Autodesk Inventor part; units mm, degrees
ref_plane "YZ Plane" through (0, 0, 0) normal (1, 0, 0) x (0, 1, 0)
ref_plane "XZ Plane" through (0, 0, 0) normal (0, 1, 0) x (-1, 0, 0)
ref_plane "XY Plane" through (0, 0, 0) normal (0, 0, 1) x (1, 0, 0)
sketch "Sketch1" plane through (0, 0, 0) normal (0, 0, 1) x (1, 0, 0)
  line L0 (-65.0875, -53.975) -> (65.0875, -53.975)
  line L1 (65.0875, -53.975) -> (65.0875, 53.975)
  line L2 (65.0875, 53.975) -> (-65.0875, 53.975)
  line L3 (-65.0875, 53.975) -> (-65.0875, -53.975)
  line L4 (-65.0875, -53.975) -> (65.0875, 53.975) construction
  line L5 (65.0875, -53.975) -> (-65.0875, 53.975) construction
  point P0 (0, 0)
  dimension "d0" = 130.175
  dimension "d1" = 107.95
extrude "Extrusion1" add sketch "Sketch1" along normal blind 209.55
sketch "Sketch2" plane through (0, 0, 209.55) normal (0, 0, 1) x (1, 0, 0)
  line L0 (-65.0875, -53.975) -> (65.0875, -53.975) construction
  line L1 (-65.0875, 53.975) -> (-65.0875, -53.975) construction
  circle A0 centre (-23.8125, -22.225) radius 4
  circle A1 centre (23.8125, 9.525) radius 4
  line L2 (-11.1125, 12.065) -> (-33.3375, 12.065)
  line L3 (-33.3375, 12.065) -> (-33.3375, 13.335)
  line L4 (-33.3375, 13.335) -> (-11.1125, 13.335)
  line L5 (-11.1125, 13.335) -> (-11.1125, 12.065)
  line L6 (-33.3375, 12.7) -> (-65.0875, 12.7) construction
  point P0 (0, 0)
  dimension "d4" = 31.75
  dimension "d5" = 41.275
  dimension "d6" = 8
  dimension "d7" = 63.5
  dimension "d8" = 88.9
  dimension "d13" = 31.75
  dimension "d14" = 53.975
  dimension "d15" = 66.675
  dimension "d16" = 1.27
extrude "Extrusion2" add sketch "Sketch2" along normal blind 12.7
sketch "Sketch3" plane through (0, 0, 0) normal (0, 0, -1) x (-1, 0, 0)
  circle A0 centre (-23.8125, 9.525) radius 4
  circle A1 centre (23.8125, -22.225) radius 4
  line L0 (33.3375, 12.065) -> (11.1125, 12.065)
  line L1 (11.1125, 12.065) -> (11.1125, 13.335)
  line L2 (11.1125, 13.335) -> (33.3375, 13.335)
  line L3 (33.3375, 13.335) -> (33.3375, 12.065)
  point P0 (0, 0)
extrude "Extrusion3" add sketch "Sketch3" along normal blind 12.7
sketch "Sketch4" plane through (-33.3375, 13.335, 0) normal (0, 1, 0) x (1, 0, 0)
  line L0 (0, 12.7) -> (22.225, 12.7)
  line L1 (22.225, 0) -> (22.225, 12.7)
  line L2 (0, 0) -> (0, 12.7)
  line L3 (22.225, -209.55) -> (22.225, -222.25)
  line L4 (22.225, -222.25) -> (0, -222.25)
  line L5 (0, -209.55) -> (0, -222.25)
  line L6 (16.51, -219.71) -> (5.715, -219.71)
  line L7 (5.715, -219.71) -> (5.715, -215.265)
  line L8 (5.715, -215.265) -> (16.51, -215.265)
  line L9 (16.51, -215.265) -> (16.51, -219.71)
  line L10 (16.51, 5.715) -> (5.715, 5.715)
  line L11 (5.715, 5.715) -> (5.715, 10.16)
  line L12 (5.715, 10.16) -> (16.51, 10.16)
  line L13 (16.51, 10.16) -> (16.51, 5.715)
  line L14 (5.715, 10.16) -> (0, 12.7) construction
  line L15 (16.51, 10.16) -> (22.225, 12.7) construction
  line L16 (22.225, -222.25) -> (16.51, -219.71) construction
  line L17 (5.715, -219.71) -> (0, -222.25) construction
  point P0 (33.3375, 0)
  dimension "d17" = 10.795
  dimension "d18" = 6.985
  dimension "d19" = 2.54
extrude "Extrusion4" cut sketch "Sketch4" against normal up to surface (1.27 mm away)
fillet "Fillet1" radius 3.175 4 edges at (-33.3375, 12.7, -12.7) (-11.1125, 12.7, -12.7) (-33.3375, 12.7, 222.25) (-11.1125, 12.7, 222.25)
thread "Thread1"
thread "Thread2"
thread "Thread3"
thread "Thread4"
sketch "Sketch5" plane through (-65.0875, 53.975, 0) normal (0, 1, 0) x (1, 0, 0)
  line L0 (25.2364, -11.8087) -> (114.825, -11.8087) construction
  line L1 (114.825, -11.8087) -> (114.825, -199.7093) construction
  line L2 (114.825, -199.7093) -> (25.2364, -199.7093) construction
  line L3 (25.2364, -199.7093) -> (25.2364, -11.8087) construction
  line L4 (91.6181, -23.1502) -> (83.0142, -23.1502)
  line L5 (83.0142, -23.1502) -> (83.0142, -31.7541)
  line L6 (83.0142, -31.7541) -> (80.1737, -31.7541)
  line L7 (80.1737, -31.7541) -> (80.1737, -23.1502)
  line L8 (80.1737, -23.1502) -> (71.5698, -23.1502)
  line L9 (71.5698, -23.1502) -> (71.5698, -20.4126)
  line L10 (71.5698, -20.4126) -> (80.1737, -20.4126)
  line L11 (80.1737, -20.4126) -> (80.1737, -11.8087)
  line L12 (80.1737, -11.8087) -> (83.0142, -11.8087)
  line L13 (83.0142, -11.8087) -> (83.0142, -20.4126)
  line L14 (83.0142, -20.4126) -> (91.6181, -20.4126)
  line L15 (91.6181, -20.4126) -> (91.6181, -23.1502)
  line L16 (33.7374, -116.5476) -> (33.7374, -94.1528)
  line L17 (33.7374, -94.1528) -> (25.2158, -94.1528)
  line L18 (25.2158, -94.1528) -> (25.2158, -91.1476)
  line L19 (25.2158, -91.1476) -> (45.6346, -91.1476)
  line L20 (45.6346, -91.1476) -> (45.6346, -94.1528)
  line L21 (45.6346, -94.1528) -> (37.1131, -94.1528)
  line L22 (37.1131, -94.1528) -> (37.1131, -116.5476)
  line L23 (37.1131, -116.5476) -> (33.7374, -116.5476)
  spline S0 degree 2 poles (66.1769, -94.0499) (67.6178, -95.7377) (69.2233, -100.6778) (69.2233, -103.8476) knots 0 0 0 1 2 2 2
  spline S1 degree 2 poles (69.2233, -103.8476) (69.2233, -106.9351) (67.6589, -111.9369) (66.1769, -113.6248) knots 0 0 0 1 2 2 2
  spline S2 degree 2 poles (66.1769, -113.6248) (64.6126, -115.3949) (60.4753, -117.0828) (57.9847, -117.0828) knots 0 0 0 1 2 2 2
  spline S3 degree 2 poles (57.9847, -117.0828) (55.4118, -117.0828) (51.2951, -115.3332) (49.7925, -113.6248) knots 0 0 0 1 2 2 2
  spline S4 degree 2 poles (49.7925, -113.6248) (48.3311, -111.9369) (46.7667, -106.9763) (46.7667, -103.8476) knots 0 0 0 1 2 2 2
  spline S5 degree 2 poles (46.7667, -103.8476) (46.7667, -100.6572) (48.3516, -95.7995) (49.8131, -94.0499) knots 0 0 0 1 2 2 2
  spline S6 degree 2 poles (49.8131, -94.0499) (51.2951, -92.362) (55.4324, -90.6125) (57.9847, -90.6125) knots 0 0 0 1 2 2 2
  spline S7 degree 2 poles (57.9847, -90.6125) (60.5782, -90.6125) (64.7361, -92.4238) (66.1769, -94.0499) knots 0 0 0 1 2 2 2
  spline S8 degree 2 poles (65.7035, -103.8476) (65.7035, -101.3364) (64.6126, -97.4462) (63.6246, -96.17) knots 0 0 0 1 2 2 2
  spline S9 degree 2 poles (63.6246, -96.17) (62.616, -94.8526) (59.7755, -93.5353) (58.0053, -93.5353) knots 0 0 0 1 2 2 2
  spline S10 degree 2 poles (58.0053, -93.5353) (56.1734, -93.5353) (53.4152, -94.8115) (52.3654, -96.17) knots 0 0 0 1 2 2 2
  spline S11 degree 2 poles (52.3654, -96.17) (51.3568, -97.4667) (50.2865, -101.3776) (50.2865, -103.8476) knots 0 0 0 1 2 2 2
  spline S12 degree 2 poles (50.2865, -103.8476) (50.2865, -108.8494) (54.4855, -114.1599) (58.0053, -114.1599) knots 0 0 0 1 2 2 2
  spline S13 degree 2 poles (58.0053, -114.1599) (61.5251, -114.1599) (65.7035, -108.8494) (65.7035, -103.8476) knots 0 0 0 1 2 2 2
  spline S14 degree 2 poles (88.9834, -98.8047) (88.9834, -100.4514) (87.8102, -103.4154) (86.7604, -104.4445) knots 0 0 0 1 2 2 2
  spline S15 degree 2 poles (86.7604, -104.4445) (85.4431, -105.7413) (81.8821, -107.0792) (79.1651, -107.0792) knots 0 0 0 1 2 2 2
  line L24 (79.1651, -107.0792) -> (76.304, -107.0792)
  line L25 (76.304, -107.0792) -> (76.304, -116.5476)
  line L26 (76.304, -116.5476) -> (72.9283, -116.5476)
  line L27 (72.9283, -116.5476) -> (72.9283, -91.1476)
  line L28 (72.9283, -91.1476) -> (79.3092, -91.1476)
  spline S16 degree 2 poles (79.3092, -91.1476) (81.5734, -91.1476) (84.7432, -91.8886) (85.9576, -92.7326) knots 0 0 0 1 2 2 2
  spline S17 degree 2 poles (85.9576, -92.7326) (87.3779, -93.7) (88.9834, -96.6846) (88.9834, -98.8047) knots 0 0 0 1 2 2 2
  spline S18 degree 2 poles (85.4636, -98.9076) (85.4636, -97.5902) (84.558, -95.6554) (83.6317, -95.0379) knots 0 0 0 1 2 2 2
  spline S19 degree 2 poles (83.6317, -95.0379) (82.829, -94.5027) (80.6883, -94.0705) (79.1034, -94.0705) knots 0 0 0 1 2 2 2
  line L29 (79.1034, -94.0705) -> (76.304, -94.0705)
  line L30 (76.304, -94.0705) -> (76.304, -104.1975)
  line L31 (76.304, -104.1975) -> (78.6093, -104.1975)
  spline S20 degree 2 poles (78.6093, -104.1975) (80.6677, -104.1975) (83.1995, -103.5389) (84.0228, -102.6744) knots 0 0 0 1 2 2 2
  spline S21 degree 2 poles (84.0228, -102.6744) (84.7844, -101.9128) (85.4636, -100.122) (85.4636, -98.9076) knots 0 0 0 1 2 2 2
  line L32 (80.0296, -190.6172) -> (70.4171, -190.6172)
  line L33 (70.4171, -190.6172) -> (70.4171, -187.5297)
  line L34 (70.4171, -187.5297) -> (80.0296, -187.5297)
  line L35 (80.0296, -187.5297) -> (80.0296, -190.6172)
  point P0 (65.0875, 0)
extrude "Extrusion7" cut sketch "Sketch5" against normal blind 0.762
sketch "Sketch6" plane through (0, 0, 0) normal (0, 0, -1) x (-1, 0, 0)
  circle A0 centre (8.3375, 46.3906) radius 3.175
  point P0 (0, 0)
  dimension "d31" = 6.35
extrude "Extrusion5" add sketch "Sketch6" along normal blind 58.42
sketch "Sketch7" plane through (-8.3375, 46.3906, -58.42) normal (0, 0, -1) x (-1, 0, 0)
  circle A0 centre (0, 0) radius 3.175
  line L0 (-16.51, -7.3025) -> (16.51, -7.3025)
  line L1 (16.51, -7.3025) -> (16.51, 7.3025)
  line L2 (16.51, 7.3025) -> (-16.51, 7.3025)
  line L3 (-16.51, 7.3025) -> (-16.51, -7.3025)
  line L4 (-16.51, -7.3025) -> (16.51, 7.3025) construction
  line L5 (16.51, -7.3025) -> (-16.51, 7.3025) construction
  point P0 (-8.3375, -46.3906)
  dimension "d34" = 14.605
  dimension "d35" = 33.02
extrude "Extrusion6" add sketch "Sketch7" along normal blind 38.1 contours A0 | L3 L2 L1 L0
properties part number "12S Module"
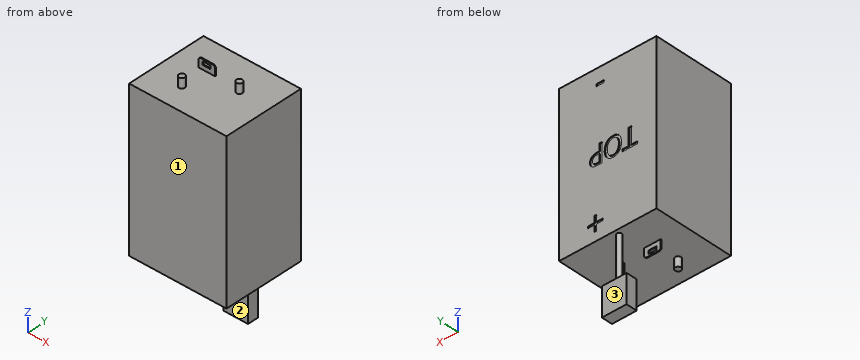
Could you check a few things on this model? Use its own coordinates, in mm. Face numbers are marked on the shaded views. A direction names the side the tool comes from. Give positions to 0.01 mm unless a question says otherwise; leave off trailing zeros. Write each loop counter-clockwise with the first axis right and the second up, starting at its lowest first coordinate (ties: lowest second). Pieces come first, ordered by that corner, then holes. Notation, with made-up numbers: (76, 39) -> (93, 39) arc R19 cw to (93, 46) -> close; hole circle Ø11 at (89.25, 72.25). An arc over 180 degrees is marked (long way). Answer as a JSON object with one key per item and string values.
Q1. Please list where these lines run through material, in increasing order: L1, parallel to Z at x = -6, y = 40; L2, parallel to Z at x = 9.5, y = -21; L3, parallel to Y at x = -7, z = -82.
Taken from the geometry:
{"L1": "z = -96.52 to -58.42, 0 to 209.55", "L2": "z = 0 to 209.55", "L3": "y = 39.09 to 53.69"}
Q2. Will these pins go through, and if not, where does the flat tip stop? pin 1 Ø1.4 at (x, y) = (-25, 12.5) entering from -Z; pin 2 Ø1 at (y, z) = (12.5, 212) entering from +X; pin 3 Ø3 at (x, z) = (-11.5, -49.5) entering from +Y.
Taken from the geometry:
{"pin 1": "stops at z = -12.7", "pin 2": "stops at x = 26.95", "pin 3": "stops at y = 49.1"}
Q3. Suppose I cut it at B-B on y = -11. Write out the boundary of the cut face in (x, z).
Taken from the geometry:
{"outline": "(-65.09, 0) -> (65.09, 0) -> (65.09, 209.55) -> (-65.09, 209.55) -> close"}
Q4. Suppose I cut it at A-A on z = -66. Write out the boundary of the cut face in (x, y), then the cut area to 3 significant figures.
Taken from the geometry:
{"outline": "(-24.85, 39.09) -> (8.17, 39.09) -> (8.17, 53.69) -> (-24.85, 53.69) -> close", "area": "482 mm²"}
Q5. Which directions (+Z, -Z, +X, -X, +Y, -Y) give clear straight access to the entire face, cutting with the end or side of a thin tool? Please do the marked faces 1, 2 and 3.
Taken from the geometry:
{"face 1": "+Z, -Z, +X, -X, -Y", "face 2": "-Z, +X, -X, -Y", "face 3": "-Z, +X, -X, +Y"}
